CAD build for the part. Positions are in the model's coordinates, mm. Round coordinates to 2 decimals unless told otherwise and drop trailing zeros. Order: outer loops, then holes, each group sorted by start corner. A loop starts at its lowest first (then second) coordinate and runs counter-clockwise, first axis right, second up. Notation, with made-up numbers: M 52.5,-17 L 71.5,-17 A21 cw 71.5,-4 Z; hole C -3.75,66 d10. An arc over 180 degrees is marked long. Answer as a JSON object with one key per item and string values.
```python
from build123d import *

# Parameters (mm, degrees)
SKETCH2_R           = 1.25
BOSS_EXTRUDE1_DEPTH = 6.5
CUT_EXTRUDE1_DEPTH  = 1


with BuildPart() as part:
    # Sketch1 → Revolve1 (revolve)
    with BuildSketch(Plane(origin=(0, 0, 0), x_dir=(0, 0, -1), z_dir=(1, 0, 0))):
        Polygon((0, 0), (-2.35, 0), (-1.25, -1.1), (-1.25, -1.5), (0, -1.5), align=None)
    revolve(axis=Axis((0, 0.872326939, 0), (0, -1, 0)))

    # Sketch2 → Boss-Extrude1 (add)
    with BuildSketch(Plane.XZ.offset(1.5)):
        Circle(SKETCH2_R)
    extrude(amount=BOSS_EXTRUDE1_DEPTH)

    # Sketch3 → Cut-Extrude1 (cut)
    with BuildSketch(Plane(origin=(0, 0, 0), x_dir=(1, 0, 0), z_dir=(0, 1, 0))):
        with BuildLine():
            Line((-1, -0.25), (-0.5, -0.25))
            ThreePointArc((-0.5, -0.25), (-0.323223305, -0.323223305), (-0.25, -0.5))
            Line((-0.25, -0.5), (-0.25, -1))
            Line((-0.25, -1), (0.25, -1))
            Line((0.25, -1), (0.25, -0.5))
            ThreePointArc((0.25, -0.5), (0.323223305, -0.323223305), (0.5, -0.25))
            Line((0.5, -0.25), (1, -0.25))
            Line((1, -0.25), (1, 0.25))
            Line((1, 0.25), (0.5, 0.25))
            ThreePointArc((0.5, 0.25), (0.323223305, 0.323223305), (0.25, 0.5))
            Line((0.25, 0.5), (0.25, 1))
            Line((0.25, 1), (-0.25, 1))
            Line((-0.25, 1), (-0.25, 0.5))
            ThreePointArc((-0.25, 0.5), (-0.323223305, 0.323223305), (-0.5, 0.25))
            Line((-0.5, 0.25), (-1, 0.25))
            Line((-1, 0.25), (-1, -0.25))
        make_face()
    extrude(amount=-CUT_EXTRUDE1_DEPTH, mode=Mode.SUBTRACT)


solid = part.part
```
Item 1: Saw through at A-A on x = 0. List the corners of the cut face in (y, z).
Worked answers:
{"outline": "M -8,-1.25 L -1.1,-1.25 L 0,-2.35 L 0,-1 L -1,-1 L -1,1 L 0,1 L 0,2.35 L -1.1,1.25 L -8,1.25 Z"}
Item 2: Saw through at C-C on y = -5.5. List the corners of the cut face in (x, z), and give its area (3 significant figures).
Worked answers:
{"outline": "C 0,0 d2.5", "area": "4.91 mm2"}
Item 3: Wall check: line 1 along Y through (x, z) = (-0.3, 0.15); line 2 along X through (y, z) = (-0.25, 0.2); line 3 along X through (y, z) = (-5, -0.4). Give the ranges that are in metal, low to high. Write a range as [from, to].
Worked answers:
{"line 1": "y = [-8, -1]", "line 2": "x = [-2.09, -1], [1, 2.09]", "line 3": "x = [-1.18, 1.18]"}
Item 4: Saw through at B-B on z = 0. List the corners of the cut face in (x, y).
Worked answers:
{"outline": "M -2.35,0 L -1.25,-1.1 L -1.25,-8 L 1.25,-8 L 1.25,-1.1 L 2.35,0 L 1,0 L 1,-1 L -1,-1 L -1,0 Z"}
Item 5: Drop flat-ended pins along their axis: pin 1 Ø0.6 at (y, z) = (-0.5, -1) entering from +X; pin 2 Ø1.5 at (x, y) = (-0.5, -2) entering from -Z; pin 3 Ø0.6 at (y, z) = (-0.5, -0.5) entering from -X; pin 4 Ø0.6 at (x, z) = (0.5, -0.5) entering from +Y. Give the stop position or say it passes through.
Worked answers:
{"pin 1": "stops at x = 1.93", "pin 2": "stops at z = -1.25", "pin 3": "stops at x = -2.1", "pin 4": "stops at y = 0"}
Item 6: Two-plate mould, pull along Z, no slides. Class faces 1 (the flat face through (0.5, 0, -0.5)), 2 (the flat face through (0, -1, 0)): released by +Z, released by -Z, zero draft, split by the parting line, or undercut.
Worked answers:
{"face 1": "zero draft", "face 2": "undercut"}
